Check sheet for the modelled part. Datum: model origin and axes. Units: mm. Round coordinates to 2 decimals unless told otherwise and drop trailing zeros. Order: outer loops, then holes, each group sorted by start corner. A loop starts at its lowest first (then second) coordinate and runs counter-clockwise, first axis right, second up. Notation, with made-up numbers: (-25, 84.5) -> (22, 84.5) arc R14 ccw to (22, 109.5) -> close; hole circle Ø11 at (40, 65.5). An arc over 180 degrees is marked (long way). Answer in a Markdown table with one row per item. Add a question column.
1. Sectioned sample at D-D, the plane y = 3. Record the boundary of the cut face in (x, z) (3 decimals), then the cut area to 3 significant figures.
2. Sectioned sample at A-A, the plane z = 0. Record the boundary of the cut face in (x, y) (3 decimals).
3. Material ranges on L1, parallel to Y at x = 8.45, z = 0 (3 decimals); L2, parallel to Z at x = 0, y = 4.2, recorded low to high. Write a range as from..to.
4. Depth check by flat-ended pin: P1, Ø1.5, axis at x = 5.5, y = 4, coming from the -Z side; P2, Ø2, axis at x = -5.5, y = 1.5, coming from the -Z side. Enter the tip coordinate at first touch or a pass-through.
5. Draft check along X on faces 1 (the flat face through (2, 6, -7)), 2 (the cylindrical face through (6.057, 2.962, -1.907)), 3 (the cylindrical face through (9.54, 2.96, -3)). Enter one of: +X half, -X half, draft (parallel to the pull), parting line (faces both ways), or undercut.
6. Sectioned sample at B-B, the plane x = 0. Record the boundary of the cut face in (y, z).
7. Sectioned sample at C-C, the plane y = 4.7. Record the boundary of the cut face in (x, z).
```python
from build123d import *

# Parameters (mm, degrees)
SKETCH1_R                = 10
SKETCH1_R_2              = 6.35
BOSS_EXTRUDE1_DEPTH      = 6
M2_5X0_45_TAPPED_HOLE1_D = 2.05
CHAMFER1_SIZE            = 0.3


with BuildPart() as part:
    # Sketch1 → Boss-Extrude1 (new body)
    with BuildSketch(Plane(origin=(0, 0, 0), x_dir=(1, 0, 0), z_dir=(0, 1, 0))):
        Circle(SKETCH1_R)
        Circle(SKETCH1_R_2, mode=Mode.SUBTRACT)
    extrude(amount=BOSS_EXTRUDE1_DEPTH)

    # M2.5x0.45 Tapped Hole1 (through all)
    with Locations(Plane(origin=(10, 0, 0), x_dir=(0, 0, -1), z_dir=(1, 0, 0))):
        with Locations((0, 3)):
            Hole(M2_5X0_45_TAPPED_HOLE1_D / 2)

    # Chamfer1
    chamfer1_edges = [part.edges().sort_by_distance(p)[0] for p in [
        (-10, 0, 0),
        (-10, 6, 0),
        (-6.35, 0, 0),
        (-6.35, 6, 0),
    ]]
    chamfer(chamfer1_edges, length=CHAMFER1_SIZE)


solid = part.part
```
Answer key:
| question | item | result |
|---|---|---|
| 1 | outline | (-9.947, -1.025) arc R10 ccw to (9.947, -1.025) -> (6.267, -1.025) arc R6.35 cw to (-6.267, -1.025) -> close; (-9.947, 1.025) -> (-6.267, 1.025) arc R6.35 cw to (6.267, 1.025) -> (9.947, 1.025) arc R10 ccw to start |
| 1 | area | 172 mm² |
| 2 | outline | (-10, 0.3) -> (-9.7, 0) -> (-6.65, 0) -> (-6.35, 0.3) -> (-6.35, 1.975) -> (-10, 1.975) -> close; (-10, 4.025) -> (-6.35, 4.025) -> (-6.35, 5.7) -> (-6.65, 6) -> (-9.7, 6) -> (-10, 5.7) -> close; (6.35, 0.3) -> (6.65, 0) -> (9.7, 0) -> (10, 0.3) -> (10, 1.975) -> (6.35, 1.975) -> close; (6.35, 4.025) -> (10, 4.025) -> (10, 5.7) -> (9.7, 6) -> (6.65, 6) -> (6.35, 5.7) -> close |
| 3 | L1 | y = 0..1.975, 4.025..6 |
| 3 | L2 | z = -10..-6.35, 6.35..10 |
| 4 | P1 | stops at z = -8.8 |
| 4 | P2 | stops at z = -8.93 |
| 5 | face 1 | draft |
| 5 | face 2 | undercut |
| 5 | face 3 | parting line |
| 6 | outline | (0, -9.7) -> (0.3, -10) -> (5.7, -10) -> (6, -9.7) -> (6, -6.65) -> (5.7, -6.35) -> (0.3, -6.35) -> (0, -6.65) -> close; (0, 6.65) -> (0.3, 6.35) -> (5.7, 6.35) -> (6, 6.65) -> (6, 9.7) -> (5.7, 10) -> (0.3, 10) -> (0, 9.7) -> close |
| 7 | outline | circle Ø20 at (0, 0); hole circle Ø12.7 at (0, 0) |
